The figure shows three views and two pictorial views of one solid part (mm, origin at its lowest corner). Answer the questions. A direction names the side the tool comes from. Give positions to 0.01 mm unless a question says otherwise; leave off trailing zeros. Write each loop counter-clockwise with the first axis right and the second up, starting at its lowest first coordinate (ties: lowest second). Pieces come first, ordered by that corner, then holes. Notation, with made-up numbers: M 82,-24.75 L 114,-24.75 A20 ccw 114,-9.75 Z; hole C 19.25,35.25 d3. An arc over 180 degrees is marked long. Return JSON: item names as keys, results as strings.
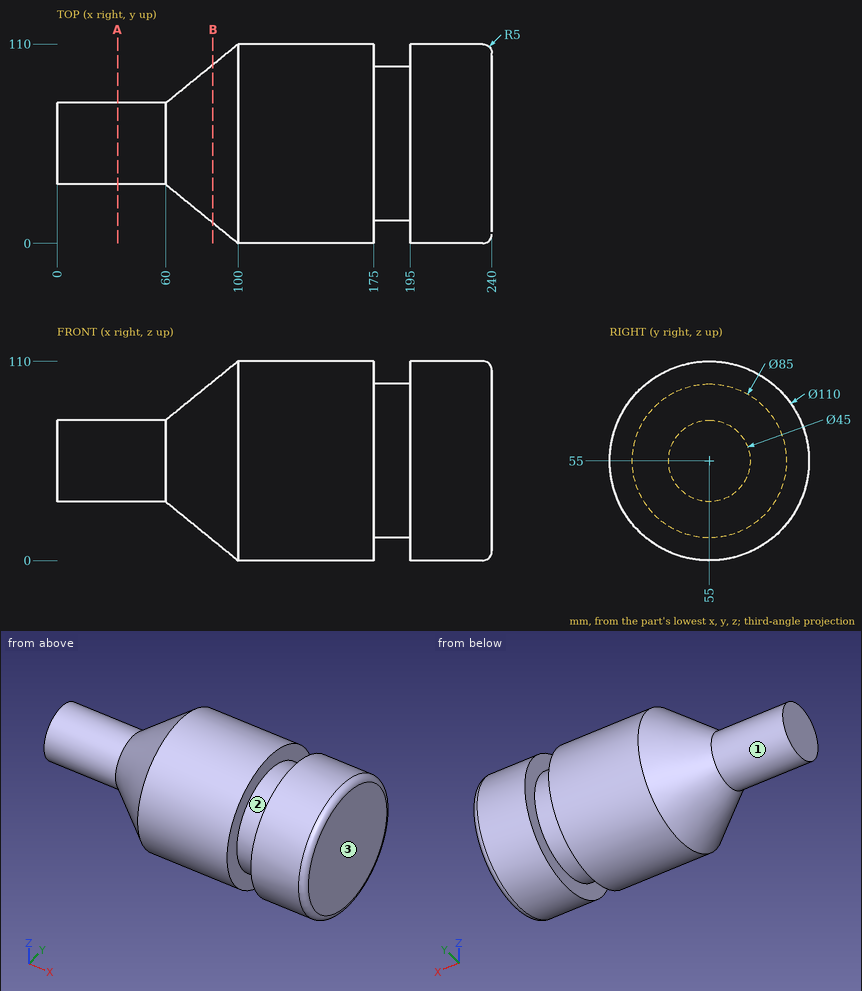
Item 1: A cutting plane is placed at B-B, the plane x = 86. Write down the section's boundary in (y, z) (3 decimals), plus the area to 3 significant figures.
Geometry results:
{"outline": "C 55,55 d87.25", "area": "5,980 mm2"}
Item 2: Given pin 1 Ø8 at (x, z) = (144, 76.5) entering from -Y; pin 2 Ø6 at (x, z) = (75, 85) entering from +Y; pin 3 Ø1.5 at (x, z) = (185.5, 83.5) entering from -Y, each flat-ended and moving along its own axis, determine where each tip first touches the part or whether it passes through.
Geometry results:
{"pin 1": "stops at y = 2.86", "pin 2": "stops at y = 78.42", "pin 3": "stops at y = 22.81"}
Item 3: Which of the six approach directions +Z, -Z, +X, -X, +Y, -Y give full straight-line access (tool end or side, diameter ignored) to the marked faces 1, 2 and 3?
Geometry results:
{"face 1": "-X", "face 2": "none", "face 3": "+Z, -Z, +X, +Y, -Y"}
Item 4: A cutting plane is placed at A-A, the plane x = 33.5. Write down the section's boundary in (y, z), plus the area to 3 significant figures.
Geometry results:
{"outline": "C 55,55 d45", "area": "1,590 mm2"}
Item 5: Find the intervals of material crossed by line 1 (X direction, y = 75.5, z = 103.5); line 2 (X direction, y = 21.5, z = 90); line 3 (Y direction, x = 93.5, z = 46), in increasing order.
Geometry results:
{"line 1": "x = 97.11 to 175, 195 to 239.24", "line 2": "x = 91.94 to 175, 195 to 240", "line 3": "y = 6.1 to 103.9"}
